from build123d import *

# Parameters (mm, degrees)
F0_W      = 128
F0_H      = 65
F1_DEPTH  = 12
F2_R      = 16
F3_R      = 26
F4_DEPTH  = 34
F5_R      = 30
F6_DEPTH  = 12
F7_R      = 15
F8_DEPTH  = 12
F9_R      = 10
F10_DEPTH = 34
F12_DEPTH = 46
F13_W     = 44
F13_H     = 8
F14_DEPTH = 46
F16_DEPTH = 25
F17_R     = 8
F18_DEPTH = 25


with BuildPart() as f1:
    # F0 (on Front) → F1 (new body)
    with BuildSketch(Plane.XZ):
        with Locations((-64, 32.5)):
            Rectangle(F0_W, F0_H)
    extrude(amount=F1_DEPTH)

    # F2
    f2_edges = [f1.edges().sort_by_distance(p)[0] for p in [
        (-128, -6, 65),
        (-128, -6, 0),
        (0, -6, 65),
        (0, -6, 0),
    ]]
    fillet(f2_edges, radius=F2_R)

    # F3 (on face) → F4 (join)
    with BuildSketch(Plane.XZ.offset(12)):
        with Locations((-64, 32.5)):
            Circle(F3_R)
    extrude(amount=F4_DEPTH)

    # F5 (on face) → F6 (join)
    with BuildSketch(Plane.XZ.offset(46)):
        with Locations((-64, 32.5)):
            Circle(F5_R)
    extrude(amount=F6_DEPTH)

    # F7 (on face) → F8 (cut)
    with BuildSketch(Plane.XZ.offset(58)):
        with Locations((-64, 32.5)):
            Circle(F7_R)
    extrude(amount=-F8_DEPTH, mode=Mode.SUBTRACT)

    # F9 (on face) → F10 (cut)
    with BuildSketch(Plane.XZ.offset(46)):
        with Locations((-64, 32.5)):
            Circle(F9_R)
    extrude(amount=-F10_DEPTH, mode=Mode.SUBTRACT)

    # F11 (on face) → F12 (cut)
    with BuildSketch(Plane.XZ.offset(58)):
        with BuildLine():
            Line((-84, 10.13932), (-84, 32.5))
            Line((-84, 32.5), (-84, 54.86068))
            ThreePointArc((-84, 54.86068), (-94, 32.5), (-84, 10.13932))
        make_face()
    extrude(amount=-F12_DEPTH, mode=Mode.SUBTRACT)

    # F13 (on face) → F14 (join)
    with BuildSketch(Plane.XZ.offset(12)):
        with Locations((-106, 32.5)):
            Rectangle(F13_W, F13_H)
    extrude(amount=F14_DEPTH)

    # F15 (on face) → F16 (cut)
    with BuildSketch(Plane(origin=(0, 0, 28.5), x_dir=(1, 0, 0), z_dir=(0, 0, -1))):
        Polygon((-128, 12), (-84, 58), (-128, 58), align=None)
    extrude(amount=-F16_DEPTH, mode=Mode.SUBTRACT)

    # F17 (on face) → F18 (cut)
    with BuildSketch(Plane.XZ.offset(12)):
        with Locations((-16, 49)):
            Circle(F17_R)
        with Locations((-16, 16)):
            Circle(F17_R)
        with Locations((-112, 49)):
            Circle(F17_R)
        with Locations((-112, 16)):
            Circle(F17_R)
    extrude(amount=-F18_DEPTH, mode=Mode.SUBTRACT)


solid = f1.part
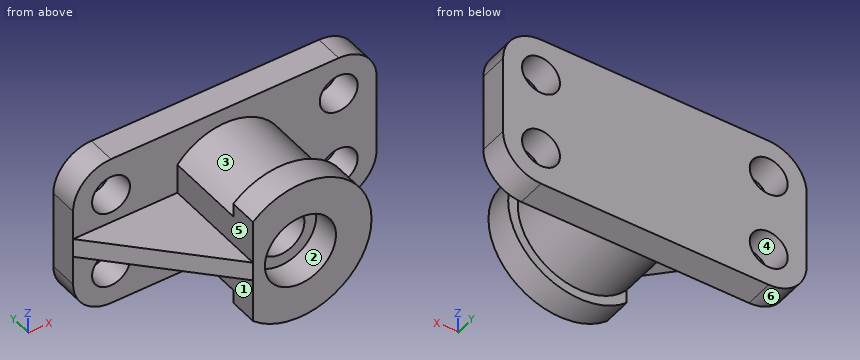
Part model, mm, in its own coordinate system. Face numbers are marked on the shaded views. A direction names the side the tool comes from. Give positions to 0.01 mm unless a question says otherwise; leave off trailing zeros. Order: outer loops, then holes, each group sorted by start corner. A loop starts at its lowest first (then second) coordinate and runs counter-clockwise, first axis right, second up. Notation, with made-up numbers: (49.25, -24.5) - (105.25, -24.5) arc R28 cw to (105.25, 14.5) - close; hole circle Ø8 at (36, 2). An arc over 180 degrees is marked (long way). Use a Markdown table: item, result.
1) Saw through at B-B on y = -5. List the corners of the cut face in (x, z).
Checked values:
| item | result |
|---|---|
| outline | (-128, 16) arc R16 ccw to (-112, 0) - (-16, 0) arc R16 ccw to (0, 16) - (0, 49) arc R16 ccw to (-16, 65) - (-112, 65) arc R16 ccw to (-128, 49) - close; hole circle Ø16 at (-112, 16); hole circle Ø16 at (-112, 49); hole circle Ø16 at (-16, 16); hole circle Ø16 at (-16, 49) |
2) Two-plate mould, pull along Z, no slides. Class the marked faces 4, 5 and 6: +Z half, -Z half, draft (parallel to the pull), parting line (faces both ways), or undercut.
Checked values:
| item | result |
|---|---|
| face 4 | undercut |
| face 5 | draft |
| face 6 | -Z half |
3) Saw through at C-C on z = 5. List the corners of the cut face in (x, y), plus the area to 3 significant figures.
Checked values:
| item | result |
|---|---|
| outline | (-123.62, -12) - (-4.38, -12) - (-4.38, 0) - (-123.62, 0) - close; (-75.99, -58) - (-52.01, -58) - (-52.01, -46) - (-75.99, -46) - close |
| area | 1,720 mm² |
4) Flat gauge pins, fed straight in: P1, Ø14.5, axis at x = -112, z = 16, coming from the +Y side (1 decimal); P2, Ø8, axis at x = -98.5, y = -34.5, coming from the +Z side; P3, Ø5.5, axis at y = -42, z = 23, coming from the -X side; P4, Ø2, axis at y = -35, z = 41.5, coming from the +X side. Where does each tip first touch, or does it go through?
Checked values:
| item | result |
|---|---|
| P1 | through |
| P2 | z = 36.5 |
| P3 | x = -84 |
| P4 | x = -39.26 |
5) Saw through at A-A on x = -13. List the corners of the cut face in (y, z).
Checked values:
| item | result |
|---|---|
| outline | (-12, 0.28) - (0, 0.28) - (0, 8.58) - (-12, 8.58) - close; (-12, 23.42) - (0, 23.42) - (0, 41.58) - (-12, 41.58) - close; (-12, 56.42) - (0, 56.42) - (0, 64.72) - (-12, 64.72) - close |
6) Probe L1, parallel to Z at x = -112, y = -7.75; L2, parallel to Z at x = -64, y = -27; L3, parallel to Z at x = -64, y = -53.25. List the from-to ranges inside material, lowest first. Write a range as from..to.
Checked values:
| item | result |
|---|---|
| L1 | 0..8, 24..41, 57..65 |
| L2 | 6.5..22.5, 42.5..58.5 |
| L3 | 2.5..17.5, 47.5..62.5 |
7) Saw through at D-D on x = -64. List the corners of the cut face in (y, z), plus the area to 3 significant figures.
Checked values:
| item | result |
|---|---|
| outline | (-58, 2.5) - (-46, 2.5) - (-46, 6.5) - (-12, 6.5) - (-12, 0) - (0, 0) - (0, 65) - (-12, 65) - (-12, 58.5) - (-46, 58.5) - (-46, 62.5) - (-58, 62.5) - (-58, 47.5) - (-46, 47.5) - (-46, 42.5) - (-12, 42.5) - (-12, 22.5) - (-46, 22.5) - (-46, 17.5) - (-58, 17.5) - close |
| area | 2,230 mm² |
8) 3-axis set-ups, long thin cutter, end or side, ignore diameter. For the marked faces 1, 2 and 3: which of +Z, -Z, +X, -X, +Y, -Y reach the whole face in a straight line?
Checked values:
| item | result |
|---|---|
| face 1 | -Z, -X, -Y |
| face 2 | -Y |
| face 3 | none |
